Work out the finished part from the listing and answer in its coordinate system (mm). Round coordinates to 2 decimals unless told otherwise and drop trailing zeros. Order: outer loops, then holes, each group sorted by start corner. A loop starts at its lowest first (then second) coordinate and runs counter-clockwise, first axis right, second up. Notation, with made-up numbers: (27.5, 29.5) - (50.5, 29.5) arc R25 cw to (50.5, 63.5) - close; hole circle Ø4 at (-4, 24). An arc over 180 degrees is marked (long way). Answer in a Markdown table with one row per item.
from build123d import *

# Parameters (mm, degrees)
SKETCH_1_R      = 5
SKETCH_1_R_2    = 2.75
EXTRUDE_1_DEPTH = 3
CHAMFER_1_SIZE  = 2.5


with BuildPart() as part:
    # Эскиз1 → Вытянуть1 (new body)
    with BuildSketch(Plane.XY):
        Polygon((-100, 190), (-92.5, 197.5), (92.5, 197.5), (100, 190), (100, -190), (92.5, -197.5), (-92.5, -197.5), (-100, -190), align=None)
        with Locations((-85, 182.5)):
            Circle(SKETCH_1_R, mode=Mode.SUBTRACT)
        with Locations(Location((85, 182.5, 0), (0, 0, 180))):
            Circle(SKETCH_1_R, mode=Mode.SUBTRACT)
        with Locations((85, -182.5)):
            Circle(SKETCH_1_R, mode=Mode.SUBTRACT)
        with Locations(Location((-85, -182.5, 0), (0, 0, 180))):
            Circle(SKETCH_1_R, mode=Mode.SUBTRACT)
        with Locations((-92.5, 150.75)):
            Circle(SKETCH_1_R_2, mode=Mode.SUBTRACT)
        with Locations(Location((-92.5, -150.75, 0), (0, 0, 180))):
            Circle(SKETCH_1_R_2, mode=Mode.SUBTRACT)
        with Locations((-92.5, 50.25)):
            Circle(SKETCH_1_R_2, mode=Mode.SUBTRACT)
        with Locations(Location((-92.5, -50.25, 0), (0, 0, 180))):
            Circle(SKETCH_1_R_2, mode=Mode.SUBTRACT)
        with Locations(Location((92.5, 150.75, 0), (0, 0, 180))):
            Circle(SKETCH_1_R_2, mode=Mode.SUBTRACT)
        with Locations(Location((92.5, 50.25, 0), (0, 0, 180))):
            Circle(SKETCH_1_R_2, mode=Mode.SUBTRACT)
        with Locations((92.5, -50.25)):
            Circle(SKETCH_1_R_2, mode=Mode.SUBTRACT)
        with Locations((92.5, -150.75)):
            Circle(SKETCH_1_R_2, mode=Mode.SUBTRACT)
    extrude(amount=EXTRUDE_1_DEPTH)

    # Фаска1
    chamfer_1_edges = [part.edges().sort_by_distance(p)[0] for p in [
        (-95.25, 150.75, 0),
        (-89.75, -150.75, 0),
        (-95.25, 50.25, 0),
        (-89.75, -50.25, 0),
        (95.25, 150.75, 0),
        (95.25, 50.25, 0),
        (89.75, -50.25, 0),
        (89.75, -150.75, 0),
    ]]
    chamfer(chamfer_1_edges, length=CHAMFER_1_SIZE)


solid = part.part
1) The mould has two halves that part along X. Classify faces 1 (the face through (84.349, -177.543, 1.479)), 2 (the face through (1, 3, 0)), 3 (the face through (-96, -194, 1)): released by +X, released by -X, zero draft, split by the parting line, or undercut.
Filled in:
| item | result |
|---|---|
| face 1 | undercut |
| face 2 | zero draft |
| face 3 | released by -X |
2) Find section A-A, the plane y = 182.5. Give the vertices of the cut face in (x, z).
Filled in:
| item | result |
|---|---|
| outline | (-100, 0) - (-90, 0) - (-90, 3) - (-100, 3) - close; (-80, 0) - (80, 0) - (80, 3) - (-80, 3) - close; (90, 0) - (100, 0) - (100, 3) - (90, 3) - close |
3) Find the intervals of material crossed by probe 1 along Y at (x, z) = (92.5, 2.85); probe 2 along X at (y, z) = (-150.75, 2.7), in increasing order. Write a range as from..to.
Filled in:
| item | result |
|---|---|
| probe 1 | y = -197.5..-153.5, -148..-53, -47.5..47.5, 53..148, 153.5..197.5 |
| probe 2 | x = -100..-95.25, -89.75..89.75, 95.25..100 |
4) Each of these flat-tipped pins is pushed along its axis until it touches: pin 1 (8 mm diameter, centred on x = -85, y = -182.5, fed in from -Z); pin 2 (6.5 mm diameter, centred on x = -92.5, y = -150.75, fed in from -Z); pin 3 (7 mm diameter, centred on x = 92.5, y = -50.25, fed in from -Z). Where does it stop, or does it pass through?
Filled in:
| item | result |
|---|---|
| pin 1 | passes through |
| pin 2 | stops at z = 2 |
| pin 3 | stops at z = 1.75 |
